CAD build for the part. Positions are in the model's coordinates, mm. Give positions to 0.01 mm unless a question says otherwise; leave off trailing zeros. Write each loop counter-clockwise with the first axis right and the second up, starting at its lowest first coordinate (ties: lowest second). Pieces come first, ordered by that corner, then holes. Notation, with made-up numbers: (7.5, 86) - (22.5, 86) arc R28 cw to (22.5, 107) - close; hole circle Ø6 at (88, 61.25). An arc over 180 degrees is marked (long way). Answer as a JSON object with one key per item and string values.
from build123d import *

# Parameters (mm, degrees)
SKETCH1_W           = 133
SKETCH1_H           = 60
SKETCH1_R           = 4
SKETCH1_R_2         = 1.75
SKETCH1_W_2         = 3
SKETCH1_H_2         = 10
SKETCH1_W_3         = 60
SKETCH1_H_3         = 20
SKETCH1_W_4         = 70
SKETCH1_H_4         = 3
BOSS_EXTRUDE2_DEPTH = 3


with BuildPart() as part:
    # Sketch1 → Boss-Extrude2 (new body)
    with BuildSketch(Plane.XY):
        Rectangle(SKETCH1_W, SKETCH1_H)
        with Locations((-51.5, -14)):
            Circle(SKETCH1_R, mode=Mode.SUBTRACT)
        with Locations((-63, 0)):
            Circle(SKETCH1_R_2, mode=Mode.SUBTRACT)
        with Locations((63, 0)):
            Circle(SKETCH1_R_2, mode=Mode.SUBTRACT)
        with Locations((63, 19)):
            Rectangle(SKETCH1_W_2, SKETCH1_H_2, mode=Mode.SUBTRACT)
        Rectangle(SKETCH1_W_3, SKETCH1_H_3, mode=Mode.SUBTRACT)
        with Locations((0, -26.5)):
            Rectangle(SKETCH1_W_4, SKETCH1_H_4, mode=Mode.SUBTRACT)
        with Locations((-63, 19)):
            Rectangle(SKETCH1_W_2, SKETCH1_H_2, mode=Mode.SUBTRACT)
        with Locations((-63, -19)):
            Rectangle(SKETCH1_W_2, SKETCH1_H_2, mode=Mode.SUBTRACT)
        with Locations((63, -19)):
            Rectangle(SKETCH1_W_2, SKETCH1_H_2, mode=Mode.SUBTRACT)
    extrude(amount=BOSS_EXTRUDE2_DEPTH)


solid = part.part
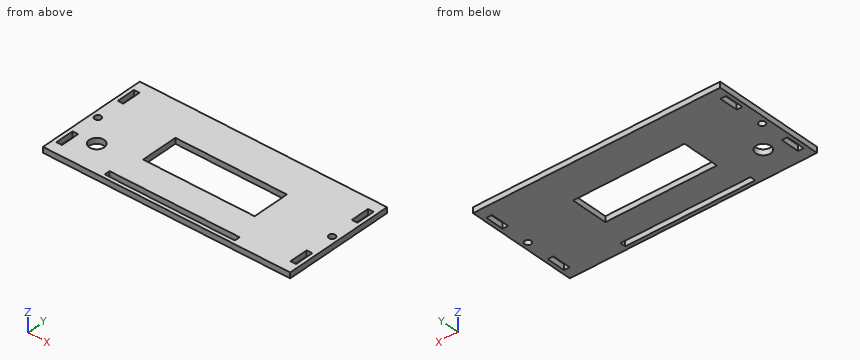
(1) Saw through at A-A, the plane x = 63. Give the cut face in (y, z), and give its area (4 significant figures).
Answer key:
{"outline": "(-30, 0) - (-24, 0) - (-24, 3) - (-30, 3) - close; (-14, 0) - (-1.75, 0) - (-1.75, 3) - (-14, 3) - close; (1.75, 0) - (14, 0) - (14, 3) - (1.75, 3) - close; (24, 0) - (30, 0) - (30, 3) - (24, 3) - close", "area": "109.5 mm²"}
(2) Saw through at C-C, the plane y = 0. Give the cut face in (x, z).
Answer key:
{"outline": "(-66.5, 0) - (-64.75, 0) - (-64.75, 3) - (-66.5, 3) - close; (-61.25, 0) - (-30, 0) - (-30, 3) - (-61.25, 3) - close; (30, 0) - (61.25, 0) - (61.25, 3) - (30, 3) - close; (64.75, 0) - (66.5, 0) - (66.5, 3) - (64.75, 3) - close"}
(3) Saw through at D-D, the plane x = 6.5. Give the cut face in (y, z).
Answer key:
{"outline": "(-30, 0) - (-28, 0) - (-28, 3) - (-30, 3) - close; (-25, 0) - (-10, 0) - (-10, 3) - (-25, 3) - close; (10, 0) - (30, 0) - (30, 3) - (10, 3) - close"}
(4) Probe L1, parallel to Y at x = -63, z = 1.3; L2, parallel to Y at x = 5.5, z = 0.35; L3, parallel to X at y = -5.5, z = 1.35. List the from-to ranges inside material, lowest first. Write a range as [from, to].
Answer key:
{"L1": "y = [-30, -24], [-14, -1.75], [1.75, 14], [24, 30]", "L2": "y = [-30, -28], [-25, -10], [10, 30]", "L3": "x = [-66.5, -30], [30, 66.5]"}
(5) Saw through at B-B, the plane z = 1.65. State how many separate pieces and enclosed holes the cut face has, and give its area (3 significant figures).
Answer key:
{"separate pieces": "1", "enclosed holes": "9", "area": "6,380 mm²"}
